```python
from build123d import *

# Parameters (mm, degrees)
F0_W     = 45.5373488367
F0_H     = 44.1119857132
F1_DEPTH = 195
F2_DEPTH = 1700
F3_DEPTH = 425
F4_T     = -60


with BuildPart() as f1:
    # F0 (on Front) → F1 (new body)
    with BuildSketch(Plane.XZ):
        with Locations((22.7686744183, 22.0559928566)):
            Rectangle(F0_W, F0_H)
    extrude(amount=F1_DEPTH)

    # F2 (add): a face of the model
    f2_faces = [f1.faces().sort_by_distance(p)[0] for p in [
        (22.7686744183, -97.5, 0),
    ]]
    extrude(f2_faces, amount=-F2_DEPTH)

    # F3 (add): a face of the model
    f3_faces = [f1.faces().sort_by_distance(p)[0] for p in [
        (0, -97.5, 850),
    ]]
    extrude(f3_faces, amount=-F3_DEPTH)

    # F4
    f4_openings = [f1.faces().sort_by_distance(p)[0] for p in [
        (212.5, -195, 850),
    ]]
    offset(amount=F4_T, openings=f4_openings)


solid = f1.part
```
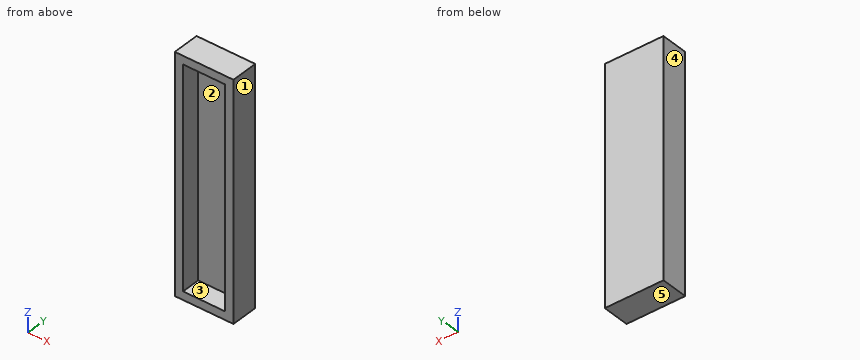
Work out the finished part from the listing and answer in its coordinate system (mm). Face numbers are marked on the shaded views. A direction names the side the tool comes from. Give positions to 0.01 mm unless a question says otherwise; leave off trailing zeros. Order: outer loops, then holes, each group sorted by start corner. A loop starts at its lowest first (then second) coordinate and runs counter-clockwise, first axis right, second up. Notation, with made-up numbers: M 85.5,18 L 127.5,18 A18 ccw 127.5,50 Z; hole C 66,44 d4. An arc over 180 degrees is marked long. Return JSON: item names as keys, results as strings.
1) Straight lines are drawn through the part: line 1 along X through (y, z) = (-103.5, 1249.5); line 2 along Z through (x, y) = (219, -156); line 3 along Y through (x, z) = (362, 280.5). For each, find the intervals that lie inside material, in ascending order. Write a range as [from, to].
Resolved:
{"line 1": "[0, 60], [365, 425]", "line 2": "[0, 60], [1640, 1700]", "line 3": "[-60, 0]"}
2) Section B-B, the plane z = 721 is taken. Write down the section's boundary in (x, y).
Resolved:
{"outline": "M 0,-195 L 60,-195 L 60,-60 L 365,-60 L 365,-195 L 425,-195 L 425,0 L 0,0 Z"}
3) This flat-tipped pin is pushed along its axis until it touches: pin 1 (5 mm diameter, centred on x = 323.5, z = 1180.5, fed in from -Y). Where does it stop, or does it pass through?
Resolved:
{"pin 1": "y = -60"}
4) A tool of negligible diameter and unlimited length cuts with its end or side. For the marked faces 1 and 2, from which of +Z, -Z, +X, -X, +Y, -Y can it reach the whole face along a straight path? Write none if from no direction.
Resolved:
{"face 1": "+Z, -Z, +X, +Y, -Y", "face 2": "-Y"}
5) Section C-C, the plane x = 132.5 is taken. Write down the section's boundary in (y, z).
Resolved:
{"outline": "M -195,0 L 0,0 L 0,1700 L -195,1700 L -195,1640 L -60,1640 L -60,60 L -195,60 Z"}
6) For a pull along Z with two mould halves and no side action, classify the marked faces 3, 4 and 5 as +Z half, -Z half, draft (parallel to the pull), parting line (faces both ways), or undercut.
Resolved:
{"face 3": "undercut", "face 4": "draft", "face 5": "-Z half"}
7) Section A-A, the plane y = -122.5 is taken. Write down the section's boundary in (x, z).
Resolved:
{"outline": "M 0,0 L 425,0 L 425,1700 L 0,1700 Z; hole M 60,60 L 365,60 L 365,1640 L 60,1640 Z"}
